from build123d import *

# Parameters (mm, degrees)
ESQUISSE1_R             = 40
BOSS_EXTRU_2_DEPTH      = 10
ESQUISSE5_R             = 5.5
ENL_V_MAT_EXTRU_2_DEPTH = 2
ESQUISSE6_R             = 15
BOSS_EXTRU_3_DEPTH      = 20
CONG_1_R                = 10
ESQUISSE7_R             = 5
ENL_V_MAT_EXTRU_3_DEPTH = 16


with BuildPart() as part:
    # Esquisse1 → Boss.-Extru.2 (new body)
    with BuildSketch(Plane.YZ):
        with Locations(Location((0, 0, 0), (0, 0, 270))):
            Circle(ESQUISSE1_R)
    extrude(amount=BOSS_EXTRU_2_DEPTH)

    # Esquisse5 → Enlèv. mat.-Extru.2 (cut)
    with BuildSketch(Plane.YZ.offset(10)):
        with Locations(Location((0, 32, 0), (0, 0, 270))):
            Circle(ESQUISSE5_R)
        with Locations(Location((12.245869836, 29.56414504, 0), (0, 0, 270))):
            Circle(ESQUISSE5_R)
        with Locations(Location((22.627416998, 22.627416998, 0), (0, 0, 270))):
            Circle(ESQUISSE5_R)
        with Locations(Location((29.56414504, 12.245869836, 0), (0, 0, 270))):
            Circle(ESQUISSE5_R)
        with Locations(Location((32, 0, 0), (0, 0, 270))):
            Circle(ESQUISSE5_R)
        with Locations(Location((29.56414504, -12.245869836, 0), (0, 0, 270))):
            Circle(ESQUISSE5_R)
        with Locations(Location((22.627416998, -22.627416998, 0), (0, 0, 270))):
            Circle(ESQUISSE5_R)
        with Locations(Location((12.245869836, -29.56414504, 0), (0, 0, 270))):
            Circle(ESQUISSE5_R)
        with Locations(Location((0, -32, 0), (0, 0, 270))):
            Circle(ESQUISSE5_R)
        with Locations(Location((-12.245869836, -29.56414504, 0), (0, 0, 270))):
            Circle(ESQUISSE5_R)
        with Locations(Location((-22.627416998, -22.627416998, 0), (0, 0, 270))):
            Circle(ESQUISSE5_R)
        with Locations(Location((-29.56414504, -12.245869836, 0), (0, 0, 270))):
            Circle(ESQUISSE5_R)
        with Locations(Location((-32, 0, 0), (0, 0, 270))):
            Circle(ESQUISSE5_R)
        with Locations(Location((-29.56414504, 12.245869836, 0), (0, 0, 270))):
            Circle(ESQUISSE5_R)
        with Locations(Location((-22.627416998, 22.627416998, 0), (0, 0, 270))):
            Circle(ESQUISSE5_R)
        with Locations(Location((-12.245869836, 29.56414504, 0), (0, 0, 270))):
            Circle(ESQUISSE5_R)
        with Locations(Location((0, 20, 0), (0, 0, 270))):
            Circle(ESQUISSE5_R)
        with Locations(Location((14.142135624, 14.142135624, 0), (0, 0, 270))):
            Circle(ESQUISSE5_R)
        with Locations(Location((20, 0, 0), (0, 0, 270))):
            Circle(ESQUISSE5_R)
        with Locations(Location((14.142135624, -14.142135624, 0), (0, 0, 270))):
            Circle(ESQUISSE5_R)
        with Locations(Location((0, -20, 0), (0, 0, 270))):
            Circle(ESQUISSE5_R)
        with Locations(Location((-14.142135624, -14.142135624, 0), (0, 0, 270))):
            Circle(ESQUISSE5_R)
        with Locations(Location((-20, 0, 0), (0, 0, 270))):
            Circle(ESQUISSE5_R)
        with Locations(Location((-14.142135624, 14.142135624, 0), (0, 0, 270))):
            Circle(ESQUISSE5_R)
        with Locations(Location((0, 8.5, 0), (0, 0, 270))):
            Circle(ESQUISSE5_R)
        with Locations(Location((8.5, 0, 0), (0, 0, 270))):
            Circle(ESQUISSE5_R)
        with Locations(Location((0, -8.5, 0), (0, 0, 270))):
            Circle(ESQUISSE5_R)
        with Locations(Location((-8.5, 0, 0), (0, 0, 270))):
            Circle(ESQUISSE5_R)
    extrude(amount=-ENL_V_MAT_EXTRU_2_DEPTH, mode=Mode.SUBTRACT)

    # Esquisse6 → Boss.-Extru.3 (add)
    with BuildSketch(Plane(origin=(0, 0, 0), x_dir=(0, -1, 0), z_dir=(-1, 0, 0))):
        with Locations(Location((0, 0, 0), (0, 0, 90))):
            Circle(ESQUISSE6_R)
    extrude(amount=BOSS_EXTRU_3_DEPTH)

    # Congé1
    cong_1_edges = [part.edges().sort_by_distance(p)[0] for p in [
        (0, 0, -15),
    ]]
    fillet(cong_1_edges, radius=CONG_1_R)

    # Esquisse7 → Enlèv. mat.-Extru.3 (cut)
    with BuildSketch(Plane.ZY.offset(20)):
        Circle(ESQUISSE7_R)
    extrude(amount=-ENL_V_MAT_EXTRU_3_DEPTH, mode=Mode.SUBTRACT)


solid = part.part
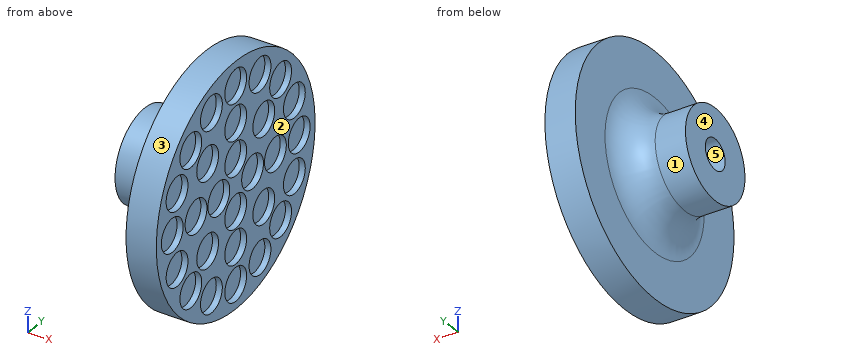
Geometry: final body of the model. Coordinates: model frame, mm. Face numbers are marked on the shaded views. A direction names the side the tool comes from. Give positions to 0.01 mm unless a question says otherwise; leave off trailing zeros. Order: outer loops, then holes, each group sorted by start corner. A loop starts at its lowest first (then second) coordinate and runs counter-clockwise, first axis right, second up. Notation, with made-up numbers: (-6, 89.25) -> (45, 89.25) arc R29 ccw to (45, 118.25) -> close; hole circle Ø2 at (-18.75, 30). An arc over 180 degrees is marked (long way). Put each result on its own line as item: value.
Q1. Section B-B, the plane z = -32. Return loops of the section in (x, y).
Here are the results:
outline: (0, -24) -> (10, -24) -> (10, -17.18) -> (8, -17.18) -> (8, -7.31) -> (10, -7.31) -> (10, -5.5) -> (8, -5.5) -> (8, 5.5) -> (10, 5.5) -> (10, 7.31) -> (8, 7.31) -> (8, 17.18) -> (10, 17.18) -> (10, 24) -> (0, 24) -> close
Q2. Section A-A, the plane x = -12.75. Return loops of the section in (y, z).
Here are the results:
outline: circle Ø30 at (0, 0); hole circle Ø10 at (0, 0)
Q3. Reachability of the marked faces 1 and 2 from +Z, -Z, +X, -X, +Y, -Y: full face, straight path, thin tool, end or side. Return the list, or none.
Here are the results:
face 1: -X
face 2: +Z, -Z, +X, +Y, -Y
Q4. Draft query along Z for the marked faces 3, 4 and 5. Return one class per face: released by +Z, released by -Z, zero draft, split by the parting line, or undercut.
Here are the results:
face 3: split by the parting line
face 4: zero draft
face 5: undercut
Q5. Pin query (flat end, axial travel): pin 1 (2 mm diameter, centred on x = -15, y = -11, fed in from +Z); pin 2 (2 mm diameter, centred on x = 3, z = 3, fed in from -Y); pin 3 (9 mm diameter, centred on y = 29.5, z = 12.5, fed in from +X). Return the tip coordinate at first contact, or that it passes through.
Here are the results:
pin 1: stops at z = 11.18
pin 2: stops at y = -39.95
pin 3: stops at x = 8
Q6. Section D-D, the plane x = 7. Return loops of the section in (y, z).
Here are the results:
outline: circle Ø80 at (0, 0)
Q7. Material intervals for L1, parallel to Y at x = 8.75, z = 8.5; L2, parallel to Z at x = 8.5, y = 32.5; L3, parallel to X at y = -35.5, z = -5.5, sorted ascending.
Here are the results:
L1: y = -39.09 to -33.59, -25.54 to -5.5, 5.5 to 25.54, 33.59 to 39.09
L2: z = -23.32 to -16.9, -7.59 to -5.48, 5.48 to 7.59, 16.9 to 23.32
L3: x = 0 to 10
